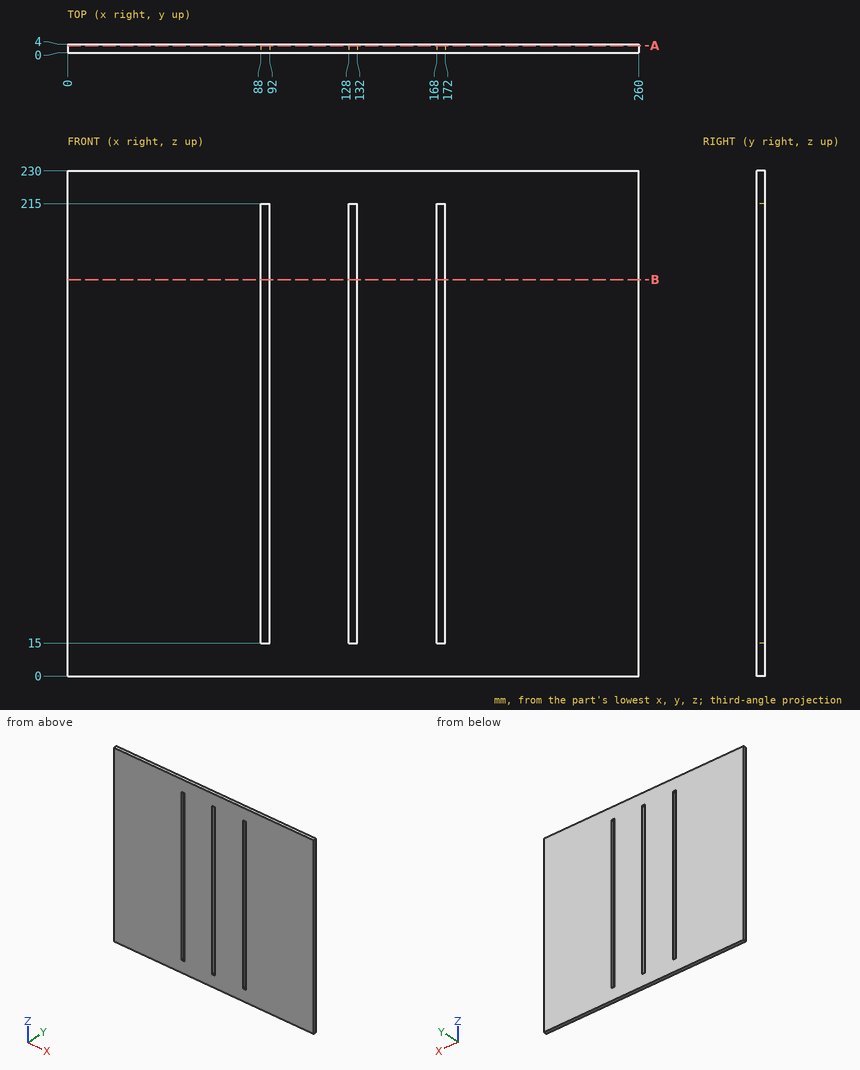
Can you work these out from the drawing? Everything is in mm from the part's minimum corner. Round coordinates to 2 decimals unless told otherwise and drop trailing zeros. Loops run counter-clockwise (first coordinate to the right, second up) from the corner with the lowest first, then second, coordinate; pieces in that order, holes last.
1. If I drill on line 1 along X through (y, z) = (0.5, 31.5); line 2 along Z through (x, y) = (129, 0.4), over which ranges is the centre line in solid material (lowest first)?
Answer list:
line 1: x = 0 to 88, 92 to 128, 132 to 168, 172 to 260
line 2: z = 0 to 15, 215 to 230
2. If we section it at B-B on z = 180.5: Write out the boundary of the cut face in (x, y).
Answer list:
outline: (0, 0) - (88, 0) - (88, 4) - (0, 4) - close; (92, 0) - (128, 0) - (128, 4) - (92, 4) - close; (132, 0) - (168, 0) - (168, 4) - (132, 4) - close; (172, 0) - (260, 0) - (260, 4) - (172, 4) - close
3. If we section it at A-A on y = 3.25: Write out the boundary of the cut face in (x, z), plus the area to 3 significant figures.
Answer list:
outline: (0, 0) - (260, 0) - (260, 230) - (0, 230) - close; hole (88, 15) - (92, 15) - (92, 215) - (88, 215) - close; hole (128, 15) - (132, 15) - (132, 215) - (128, 215) - close; hole (168, 15) - (172, 15) - (172, 215) - (168, 215) - close
area: 57,400 mm2
